The listing builds one solid part. Answer for the finished solid, in the listing's coordinates (mm). Face numbers are marked on the shaded views. A direction names the side the tool comes from. Coordinates: 2 decimals unless noted, no trailing zeros. Order: outer loops, then holes, each group sorted by start corner. A loop starts at its lowest first (then second) coordinate and runs counter-clockwise, first axis right, second up. Notation, with made-up numbers: M -13,89.25 L 10,89.25 A28 ccw 10,117.25 Z; hole C -24.75,13.25 d8. An arc over 180 degrees is marked long. One line per item, written item: value. Start each with the question number.
Q1. The part is cut by section A-A on y = 3.6. Give the vertices of the cut face in (x, z).
Q2. For the marked faces 4, 5, 6 and 7, determine the directions among +Z, -Z, +X, -X, +Y, -Y from which every point of the face is accessible in a straight line to the end or side of a thin tool.
Q3. Determine the mould class of the marked faces 1, 2 and 3 for opening direction X: pulls with the +X half, pulls with the -X half, needs draft (parallel to the pull), parting line crosses it, or undercut.
Q4. The part is cut by section C-C on z = -2.75. Give the vertices of the cut face in (x, y).
Q5. Each of these flat-tipped pins is pushed along its axis until it touches: pin 1 Ø1.7 at (y, z) = (2, -3.5) entering from -X; pin 2 Ø1.5 at (x, y) = (5, 2.5) entering from -Z. Where does it stop, or does it pass through?
Q6. The part is cut by section B-B on x = 2.5. Give the vertices of the cut face in (y, z).
Q7. The part is cut by section D-D on y = 0.3. Give the vertices of the cut face in (x, z).
Q8. Straight lines are drawn through the part: line 1 along Y through (x, z) = (-2.25, -5.25); line 2 along X through (y, z) = (1.35, 2); line 3 along X through (y, z) = (4, -4.5). For each, find the intervals that lie inside material, in ascending order. Write a range as [from, to].
Autodesk Inventor part; units mm, degrees
ref_plane "YZ Plane" through (0, 0, 0) normal (1, 0, 0) x (0, 1, 0)
ref_plane "XZ Plane" through (0, 0, 0) normal (0, 1, 0) x (-1, 0, 0)
ref_plane "XY Plane" through (0, 0, 0) normal (0, 0, 1) x (1, 0, 0)
sketch "Szkic1" plane through (0, 0, 0) normal (0, 1, 0) x (-1, 0, 0)
  line L0 (4.0644, 4.4067) -> (-5.7356, 4.4067)
  line L1 (-5.7356, 4.4067) -> (-5.7356, -5.3933)
  line L2 (-5.7356, -5.3933) -> (4.0644, -5.3933)
  line L3 (4.0644, -5.3933) -> (4.0644, 4.4067)
  line L4 (4.0644, 4.4067) -> (-5.7356, -5.3933) construction
  line L5 (-5.7356, 4.4067) -> (4.0644, -5.3933) construction
  line L6 (-0.8356, -0.4933) -> (-0.8356, -4.9033)
  line L7 (-0.8356, -0.4933) -> (-5.2456, -0.4933)
  line L8 (-5.2456, -0.4933) -> (-0.8356, -4.9033)
  line L9 (-0.8356, -0.4933) -> (-1.796, -0.4933)
  line L10 (-0.8356, -0.4933) -> (2.5944, -0.4933)
  line L11 (-0.8356, -0.4933) -> (2.5944, -0.4933) construction
  line L12 (2.5944, -0.4933) -> (2.5944, -4.9033)
  line L13 (2.5944, -4.9033) -> (-1.796, -0.4933)
  line L14 (-5.2456, -0.4933) -> (-0.8356, 3.9167)
  line L15 (2.5944, 3.9167) -> (-1.796, -0.4933)
  line L16 (2.5944, -0.4933) -> (2.5944, 3.9167)
  line L17 (-0.8356, -0.4933) -> (-0.8356, 3.9167)
  line L18 (-6.7156, 5.3867) -> (5.0444, 5.3867)
  line L19 (5.0444, 5.3867) -> (5.0444, -6.3733)
  line L20 (5.0444, -6.3733) -> (-6.7156, -6.3733)
  line L21 (-6.7156, -6.3733) -> (-6.7156, 5.3867)
  line L22 (-6.7156, 5.3867) -> (5.0444, -6.3733) construction
  line L23 (5.0444, 5.3867) -> (-6.7156, -6.3733) construction
  point P0 (0, 0)
  point P1 (-0.8356, -1.458)
  point P2 (-0.8356, 0.4714)
  dimension "d0" = 9.8
  dimension "d1" = 9.8
  dimension "d2" = 4.41
  dimension "d3" = 4.41
  dimension "d4" = 0.9604
  dimension "d5" = 3.43
  dimension "d6" = 0
  dimension "d7" = 4.41
  dimension "d8" = 90
  dimension "d9" = 11.76
  dimension "d10" = 11.76
extrude "Wyciągnięcie proste1" add sketch "Szkic1" along normal blind 0.5 contours L3 L2 L1 L0 | L10 L12 L13 L6 | L6 L13 L7 | L17 L15 L16 L10 | L7 L15 L17 | L6 L8 L7 L13 | L7 L14 L17 L15 | L18 L19 L20 L21
extrude "Wyciągnięcie proste2" add sketch "Szkic1" along normal blind 5 contours L10 L12 L13 L6 | L6 L13 L7 | L17 L15 L16 L10 | L7 L15 L17 | L6 L8 L7 L13 | L7 L14 L17 L15
fillet "Zaokrąglenie1" radius 2 4 edges at (6.7156, 0.25, 5.3867) (-5.0444, 0.25, 5.3867) (6.7156, 0.25, -6.3733) (-5.0444, 0.25, -6.3733)
offset faces "Rozmiar1" outward -0.04 faces at (2.3056, 2, 2.4467) (-1.4511, 2, 2.7682) (3.7756, 2, -1.9633) (0.8356, 2, -3.7549) (-0.3078, 2, -2.6064) (-2.5944, 3.5, -1.9633)
properties part number "guzik_musik"
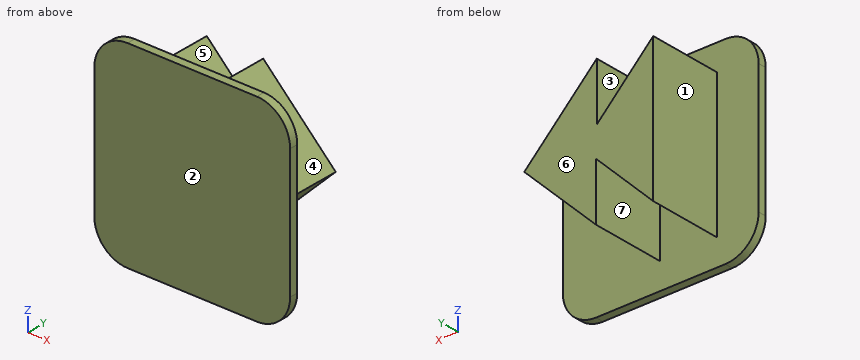
Output:
1. outline: M -2.55,-4.81 L 0.88,-1.36 L 0.88,-4.81 L 5.19,-0.49 L 0.84,3.86 L 0.84,0.41 L -2.55,3.82 Z
2. face 4: +Z, +X, +Y
2. face 5: +Z, +Y
2. face 6: +Z, -Z, +X, -X, +Y
2. face 7: -Z, +Y
3. face 1: pulls with the -X half
3. face 2: needs draft
3. face 3: undercut
4. outline: M -5.04,0 L 6.72,0 L 6.72,0.5 L 2.93,0.5 L 2.93,5 L 0.88,5 L 0.88,0.5 L -0.51,0.5 L -0.51,5 L -2.55,5 L -2.55,0.5 L -5.04,0.5 Z
5. pin 1: stops at x = -2.55
5. pin 2: stops at z = -1.43
6. outline: M 0,-6.37 L 0.5,-6.37 L 0.5,-3.18 L 5,-3.18 L 5,2.2 L 0.5,2.2 L 0.5,5.39 L 0,5.39 Z
7. outline: M -5.04,-4.37 A2 ccw -3.04,-6.37 L 4.72,-6.37 A2 ccw 6.72,-4.37 L 6.72,3.39 A2 ccw 4.72,5.39 L -3.04,5.39 A2 ccw -5.04,3.39 Z
8. line 1: y = [0, 0.5]
8. line 2: x = [-2.55, -0.74], [0.84, 2.7]
8. line 3: x = [-2.55, -2.25], [0.88, 1.18]
